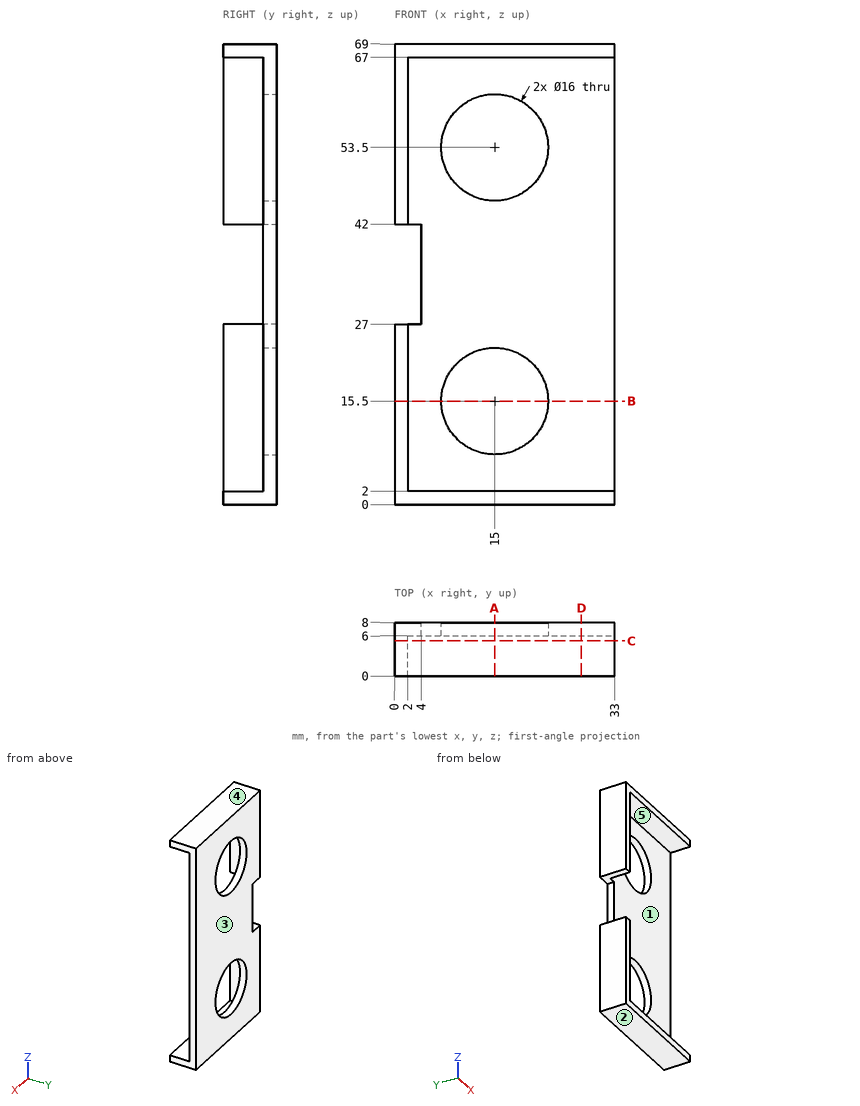
The drawing under review shows one solid part. Ordinate dimensions are in mm from its lowest x, y, z. A direction names the side the tool comes from. Round coordinates to 2 decimals unless told otherwise and drop trailing zeros. Write each loop counter-clockwise with the first axis right and the second up, starting at its lowest first coordinate (ties: lowest second). Pieces come first, ordered by that corner, then holes. Notation, with made-up numbers: (69.25, 59.5) -> (110.25, 59.5) arc R9 ccw to (110.25, 65.5) -> close; hole circle Ø1 at (24, -25.5). An arc over 180 degrees is marked (long way). Put each result on its own line as item: value.
Q1. Consider section A-A on x = 15. State the section outline as (y, z) points.
Determined:
outline: (0, 0) -> (8, 0) -> (8, 7.5) -> (6, 7.5) -> (6, 2) -> (0, 2) -> close; (0, 67) -> (6, 67) -> (6, 61.5) -> (8, 61.5) -> (8, 69) -> (0, 69) -> close; (6, 23.5) -> (8, 23.5) -> (8, 45.5) -> (6, 45.5) -> close
Q2. Consider section C-C on y = 5.25. State the section outline as (x, z) points, and give its area (3 significant figures).
Determined:
outline: (0, 0) -> (33, 0) -> (33, 2) -> (2, 2) -> (2, 27) -> (0, 27) -> close; (0, 42) -> (2, 42) -> (2, 67) -> (33, 67) -> (33, 69) -> (0, 69) -> close
area: 232 mm^2
Q3. Machinability: for the marked faces 4 and 5, which of the approach directions +Z, -Z, +X, -X, +Y, -Y give a long, thin tool a straight path to every point of the face, cutting with its end or side? Answer none if there is none.
Determined:
face 4: +Z, +X, -X, +Y, -Y
face 5: +X, -Y
Q4. Consider section D-D on x = 28. State the section outline as (y, z) points.
Determined:
outline: (0, 0) -> (8, 0) -> (8, 69) -> (0, 69) -> (0, 67) -> (6, 67) -> (6, 2) -> (0, 2) -> close
Q5. To check wall thickness, follow L1, parallel to Z at x = 15, y = 7.65; L2, parallel to Z at x = 6.5, y = 5.5; L3, parallel to Z at x = 13, y = 6.5. State the ranges of each line that lie inside material, in increasing order. Write a range as [from, to].
Determined:
L1: z = [0, 7.5], [23.5, 45.5], [61.5, 69]
L2: z = [0, 2], [67, 69]
L3: z = [0, 7.75], [23.25, 45.75], [61.25, 69]
Q6. Clearance check with flat-ended pins moving along their axes: pin 1 Ø18.5 at (x, z) = (15, 53.5) entering from -Y; pin 2 Ø1.6 at (y, z) = (7.5, 37) entering from -X. State where each tip first meets the part, or that it passes through.
Determined:
pin 1: stops at y = 6
pin 2: stops at x = 4
Q7. The part is to be moulded in two halves that separate along Z. For the marked faces 1, 2 and 3, say which applies: released by +Z, released by -Z, zero draft, split by the parting line, or undercut.
Determined:
face 1: undercut
face 2: released by -Z
face 3: zero draft
Q8. Consider section B-B on z = 15.5. State the section outline as (x, y) points, and give its area (3 significant figures).
Determined:
outline: (0, 0) -> (2, 0) -> (2, 6) -> (7, 6) -> (7, 8) -> (0, 8) -> close; (23, 6) -> (33, 6) -> (33, 8) -> (23, 8) -> close
area: 46.0 mm^2
